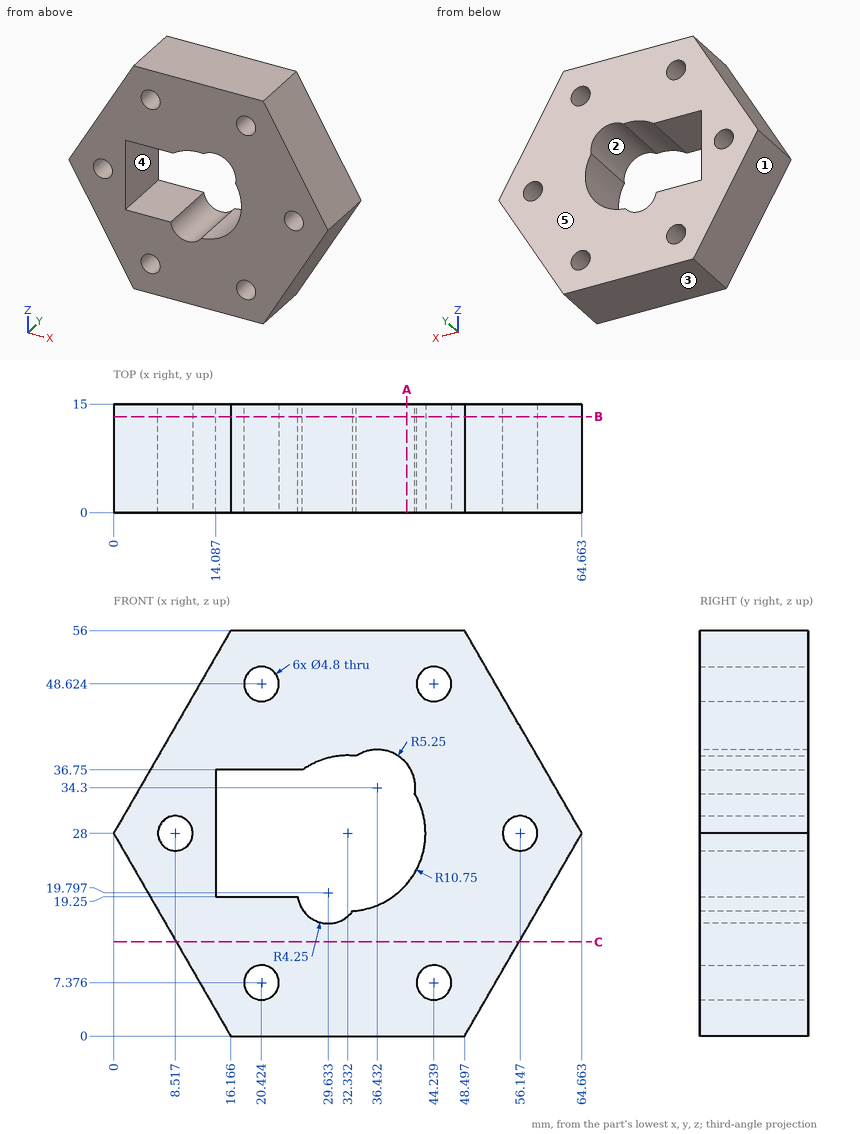
Check sheet for the drawn part. Datum: minimum x, y, z corner. Units: mm. A direction names the side the tool comes from. Round coordinates to 2 decimals unless told otherwise and drop trailing zeros. Order: outer loops, then holes, each group sorted by start corner. A loop starts at its lowest first (then second) coordinate and runs counter-clockwise, first axis right, second up. Notation, with made-up numbers: (-7.5, -18) -> (9.5, -18) arc R23 ccw to (9.5, 0) -> close; hole circle Ø5 at (21.25, 63). An arc over 180 degrees is marked (long way). Return JSON: item names as keys, results as strings. Group by question number.
Q1. Section check C-C, the plane z = 13. Record the boundary of the cut face in (x, y).
Q2. Material ranges on probe 1 along Z at (x, y) = (23, 3); probe 2 along X at (y, z) = (8.75, 7.5) (1 decimal); probe 3 along X at (y, z) = (2.5, 46.5) (1 decimal), recorded low to high. Write a range as from..to.
Q3. Section check A-A, the plane x = 40.5. Record the boundary of the cut face in (y, z), plus the area to 3 significant figures.
Q4. Tool access check on the marked faces 4 and 5. Record the directions out of +Z, -Z, +X, -X, +Y, -Y that give a thin tool (end or side, any length) a straight path to the whole face; none if there is none.
Q5. Gauge pin test, flat ends, axial feed: pin 1 (7.5 mm diameter, centred on y = 11, z = 29, fed in from +X); pin 2 (4 mm diameter, centred on x = 44.24, z = 48.62, fed in from +Y); pin 3 (1.5 mm diameter, centred on y = 9, z = 50, fed in from -X); pin 4 (8 mm diameter, centred on y = 6.5, z = 33.5, fed in from -X) (1 decimal). Record the tip position at first contact, or that the pin passes through.
Q6. Release check for a two-part mould opening along X. For the marked faces 1, 2 and 3 record: released by +X, released by -X, zero draft, split by the parting line, or undercut.
Q7. Section check B-B, the plane y = 13.25. Count the separate pieces of the cut face and the enclosed holes in it, plus the area to 3 significant figures.
Numbers:
{
 "1": {"outline": "(8.66, 0) -> (56, 0) -> (56, 15) -> (8.66, 15) -> close"},
 "2": {"probe 1": "0..19.25, 36.75..56", "probe 2": "11.8..18, 22.8..41.8, 46.6..52.8", "probe 3": "10.7..19.3, 21.5..43.1, 45.4..54"},
 "3": {"outline": "(0, 0) -> (15, 0) -> (15, 21.01) -> (0, 21.01) -> close; (0, 37.62) -> (15, 37.62) -> (15, 56) -> (0, 56) -> close", "area": "591 mm^2"},
 "4": {"face 4": "+Y, -Y", "face 5": "+Z, -Z, +X, -X, +Y"},
 "5": {"pin 1": "x = 64.66", "pin 2": "through", "pin 3": "x = 12.27", "pin 4": "x = 0.9"},
 "6": {"face 1": "released by -X", "face 2": "undercut", "face 3": "zero draft"},
 "7": {"separate pieces": "1", "enclosed holes": "7", "area": "2,060 mm^2"}
}
